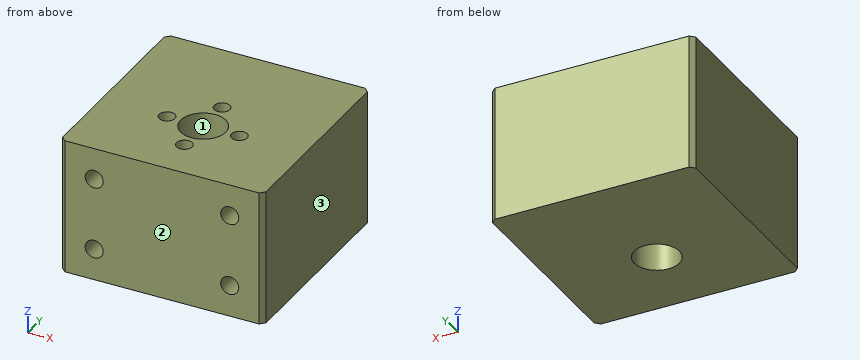
from build123d import *

# Parameters (mm, degrees)
SKETCH1_W           = 45
SKETCH1_H           = 45
SKETCH1_R           = 5
BOSS_EXTRUDE1_DEPTH = 15
SKETCH2_R           = 1.75
CUT_EXTRUDE1_DEPTH  = 10
CHAMFER1_SIZE       = 1
SKETCH3_R           = 2
CUT_EXTRUDE2_DEPTH  = 10


with BuildPart() as part:
    # Sketch1 → Boss-Extrude1 (new body, symmetric)
    with BuildSketch(Plane.XY):
        with Locations((0, 5)):
            Rectangle(SKETCH1_W, SKETCH1_H)
        Circle(SKETCH1_R, mode=Mode.SUBTRACT)
    extrude(amount=BOSS_EXTRUDE1_DEPTH, both=True)

    # Sketch2 → Cut-Extrude1 (cut)
    with BuildSketch(Plane.XY.offset(15)):
        with Locations((0, 8)):
            Circle(SKETCH2_R)
        with Locations((0, -8)):
            Circle(SKETCH2_R)
        with Locations((8, 0)):
            Circle(SKETCH2_R)
        with Locations((-8, 0)):
            Circle(SKETCH2_R)
    extrude(amount=-CUT_EXTRUDE1_DEPTH, mode=Mode.SUBTRACT)

    # Chamfer1
    chamfer1_edges = [part.edges().sort_by_distance(p)[0] for p in [
        (-22.5, 27.5, 0),
        (22.5, 27.5, 0),
        (22.5, -17.5, 0),
        (-22.5, -17.5, 0),
    ]]
    chamfer(chamfer1_edges, length=CHAMFER1_SIZE)

    # Sketch3 → Cut-Extrude2 (cut)
    with BuildSketch(Plane.XZ.offset(17.5)):
        with Locations((15, 8)):
            Circle(SKETCH3_R)
        with Locations((15, -8)):
            Circle(SKETCH3_R)
    cut_extrude2 = extrude(amount=-CUT_EXTRUDE2_DEPTH, mode=Mode.SUBTRACT)

    # Mirror1: Cut-Extrude2 across plane
    add(cut_extrude2.mirror(Plane(origin=(0, 0, 0), x_dir=(0, 0, 1), z_dir=(1, 0, 0))), mode=Mode.SUBTRACT)


solid = part.part
Could you check a few things on this model? Use its own coordinates, in mm. Face numbers are marked on the shaded views. Round coordinates to 2 decimals unless told otherwise and drop trailing zeros. Order: outer loops, then holes, each group sorted by start corner. A loop starts at its lowest first (then second) coordinate and runs counter-clockwise, first axis right, second up.
Q1. Imagine slicing it at D-D, the plane x = -15. List the corners of the cut face in (y, z) for me, then the cut area to 3 significant figures.
Geometry says:
outline: (-17.5, -15) - (27.5, -15) - (27.5, 15) - (-17.5, 15) - (-17.5, 10) - (-7.5, 10) - (-7.5, 6) - (-17.5, 6) - (-17.5, -6) - (-7.5, -6) - (-7.5, -10) - (-17.5, -10) - close
area: 1,270 mm2
Q2. I'm going to push flat-ended pins straight in: P1, Ø12, axis at x = -4, y = -0.5, coming from the +Z side; P2, Ø1.2, axis at x = -15.5, z = 7.5, coming from the -Y side; P3, Ø1.8, axis at x = 0.5, y = -8.5, coming from the +Z side. Where does each tip first touch, or does it pass through?
Geometry says:
P1: stops at z = 15
P2: stops at y = -7.5
P3: stops at z = 5
Q3. Imagine slicing it at B-B, the plane x = 3. List the corners of the cut face in (y, z) for me, then the cut area to 3 significant figures.
Geometry says:
outline: (-17.5, -15) - (-4, -15) - (-4, 15) - (-17.5, 15) - close; (4, -15) - (27.5, -15) - (27.5, 15) - (4, 15) - close
area: 1,110 mm2
Q4. Thinking about a two-plate mould opening in X: for the marked faces 1, 2 and 3, which applies, released by +X, released by -X, zero draft, split by the parting line, or undercut?
Geometry says:
face 1: undercut
face 2: zero draft
face 3: released by +X
Q5. Imagine slicing it at A-A, the plane y = 0. List the corners of the cut face in (x, z) for me, then the cut area to 3 significant figures.
Geometry says:
outline: (-22.5, -15) - (-5, -15) - (-5, 15) - (-6.25, 15) - (-6.25, 5) - (-9.75, 5) - (-9.75, 15) - (-22.5, 15) - close; (5, -15) - (22.5, -15) - (22.5, 15) - (9.75, 15) - (9.75, 5) - (6.25, 5) - (6.25, 15) - (5, 15) - close
area: 980 mm2
Q6. Please list where these lines run through material, in increasing order: probe 1 along Y at (x, z) = (0, 12.5); probe 2 along Y at (x, z) = (0, -3); probe 3 along Y at (x, z) = (6.5, 5.25).
Geometry says:
probe 1: y = -17.5 to -9.75, -6.25 to -5, 5 to 6.25, 9.75 to 27.5
probe 2: y = -17.5 to -5, 5 to 27.5
probe 3: y = -17.5 to -0.9, 0.9 to 27.5
Q7. Imagine slicing it at C-C, the plane z = 3.75. List the corners of the cut face in (x, y) for me.
Geometry says:
outline: (-22.5, -16.5) - (-21.5, -17.5) - (21.5, -17.5) - (22.5, -16.5) - (22.5, 26.5) - (21.5, 27.5) - (-21.5, 27.5) - (-22.5, 26.5) - close; hole circle Ø10 at (0, 0)
